The model under review builds one solid part; all positions refer to its coordinate system, in mm. A direction names the side the tool comes from. Round coordinates to 2 decimals unless told otherwise and drop trailing zeros. Write each loop counter-clockwise with the first axis right and the second up, starting at its lowest first coordinate (ties: lowest second). Pieces come first, ordered by that corner, then holes. Notation, with made-up numbers: (62, 6) -> (84, 6) arc R25 cw to (84, 39) -> close; hole circle Ø4 at (87.25, 70). An arc over 180 degrees is marked (long way). Answer in a Markdown table with one row per item. Add a question column.
Autodesk Inventor part; units mm, degrees
ref_plane "YZ Plane" through (0, 0, 0) normal (1, 0, 0) x (0, 1, 0)
ref_plane "XZ Plane" through (0, 0, 0) normal (0, 1, 0) x (-1, 0, 0)
ref_plane "XY Plane" through (0, 0, 0) normal (0, 0, 1) x (1, 0, 0)
sketch "Sketch1" plane through (0, 0, 0) normal (0, 1, 0) x (-1, 0, 0)
  line L0 (0, 0) -> (152.4, 0)
  line L1 (152.4, 0) -> (152.4, 152.4)
  line L2 (152.4, 152.4) -> (0, 152.4)
  line L3 (0, 152.4) -> (0, 0)
  dimension "d0" = 152.4
  dimension "d1" = 152.4
extrude "Extrusion1" add sketch "Sketch1" along normal blind 6.35
sketch "Sketch2" plane through (0, 6.35, 0) normal (0, 1, 0) x (1, 0, 0)
  line L0 (-142.24, -142.24) -> (-77.47, -142.24)
  line L1 (-77.47, -142.24) -> (-77.47, -132.08)
  line L2 (-77.47, -132.08) -> (-142.24, -132.08)
  line L3 (-142.24, -132.08) -> (-142.24, -142.24)
  line L4 (-74.93, -142.24) -> (-10.16, -142.24)
  line L5 (-10.16, -142.24) -> (-10.16, -132.08)
  line L6 (-10.16, -132.08) -> (-74.93, -132.08)
  line L7 (-74.93, -132.08) -> (-74.93, -142.24)
  line L8 (-152.4, 0) -> (-152.4, -152.4)
  line L9 (-152.4, -152.4) -> (0, -152.4)
  line L10 (0, -152.4) -> (0, 0)
  line L11 (-152.4, -76.2) -> (0, -76.2) construction
  line L12 (-142.24, -10.16) -> (-77.47, -10.16)
  line L13 (-77.47, -10.16) -> (-77.47, -20.32)
  line L14 (-77.47, -20.32) -> (-142.24, -20.32)
  line L15 (-142.24, -20.32) -> (-142.24, -10.16)
  line L16 (-74.93, -10.16) -> (-10.16, -10.16)
  line L17 (-10.16, -10.16) -> (-10.16, -20.32)
  line L18 (-10.16, -20.32) -> (-74.93, -20.32)
  line L19 (-74.93, -20.32) -> (-74.93, -10.16)
  point P0 (-10.16, -137.16)
  point P1 (-10.16, -15.24)
  dimension "d4" = 10.16
  dimension "d5" = 10.16
  dimension "d6" = 10.16
  dimension "d7" = 64.77
  dimension "d8" = 64.77
  dimension "d9" = 10.16
  dimension "d10" = 10.16
  dimension "d11" = 10.16
extrude "Extrusion2" cut sketch "Sketch2" against normal through all
sketch "Sketch3" plane through (0, 6.35, 0) normal (0, 1, 0) x (1, 0, 0)
  line L0 (-77.47, -20.32) -> (-142.24, -20.32)
  line L1 (-142.24, -20.32) -> (-142.24, -10.16)
  line L2 (-142.24, -10.16) -> (-77.47, -10.16)
  line L3 (-77.47, -10.16) -> (-77.47, -20.32)
  line L4 (-74.93, -132.08) -> (-10.16, -132.08)
  line L5 (-10.16, -132.08) -> (-10.16, -142.24)
  line L6 (-10.16, -142.24) -> (-74.93, -142.24)
  line L7 (-74.93, -142.24) -> (-74.93, -132.08)
  line L8 (-10.16, -10.16) -> (-10.16, -20.32)
  line L9 (-10.16, -20.32) -> (-74.93, -20.32)
  line L10 (-74.93, -20.32) -> (-74.93, -10.16)
  line L11 (-74.93, -10.16) -> (-10.16, -10.16)
  line L12 (-142.24, -132.08) -> (-77.47, -132.08)
  line L13 (-77.47, -132.08) -> (-77.47, -142.24)
  line L14 (-77.47, -142.24) -> (-142.24, -142.24)
  line L15 (-142.24, -142.24) -> (-142.24, -132.08)
  line L16 (-152.4, 0) -> (-152.4, -152.4)
  line L17 (-152.4, -152.4) -> (0, -152.4)
  line L18 (0, -152.4) -> (0, 0)
  line L19 (0, 0) -> (-152.4, 0)
  line L20 (-146.05, -146.05) -> (-146.05, -6.35)
  line L21 (-146.05, -6.35) -> (-6.35, -6.35)
  line L22 (-6.35, -6.35) -> (-6.35, -146.05)
  line L23 (-6.35, -146.05) -> (-146.05, -146.05)
  dimension "d14" = 6.35
extrude "Extrusion3" add sketch "Sketch3" along normal blind 38.1 contours L19 L18 L17 L16
ref_plane "Work Plane1" through (0, 22.225, 0) normal (0, 1, 0) x (1, 0, 0)
mirror "Mirror1" about plane through (0, 22.225, 0) normal (0, 1, 0) of "Extrusion1", "Extrusion2"
sketch "Sketch5" plane through (0, 22.225, 0) normal (0, 1, 0) x (1, 0, 0)
  line L0 (-142.24, -10.16) -> (-77.47, -10.16)
  line L1 (-77.47, -10.16) -> (-77.47, -20.32)
  line L2 (-77.47, -20.32) -> (-142.24, -20.32)
  line L3 (-142.24, -20.32) -> (-142.24, -10.16)
  line L4 (-142.24, -142.24) -> (-142.24, -132.08)
  line L5 (-142.24, -132.08) -> (-77.47, -132.08)
  line L6 (-77.47, -132.08) -> (-77.47, -142.24)
  line L7 (-77.47, -142.24) -> (-142.24, -142.24)
  line L8 (-74.93, -20.32) -> (-74.93, -10.16)
  line L9 (-74.93, -10.16) -> (-10.16, -10.16)
  line L10 (-10.16, -10.16) -> (-10.16, -20.32)
  line L11 (-10.16, -20.32) -> (-74.93, -20.32)
  line L12 (-74.93, -142.24) -> (-74.93, -132.08)
  line L13 (-74.93, -132.08) -> (-10.16, -132.08)
  line L14 (-10.16, -132.08) -> (-10.16, -142.24)
  line L15 (-10.16, -142.24) -> (-74.93, -142.24)
  line L16 (-152.4, -152.4) -> (0, -152.4)
  line L17 (0, -152.4) -> (0, 0)
  line L18 (0, 0) -> (-152.4, 0)
  line L19 (-152.4, 0) -> (-152.4, -152.4)
extrude "Extrusion4" cut sketch "Sketch5" against normal through all contours L0 L1 L2 L3 | L4 L5 L6 L7 | L8 L9 L10 L11 | L12 L13 L14 L15 | L19 L18 L17 L16
equation "\"d8\" = d7"
equation "\"d10\" = d5"
equation "\"d11\" = d6"
properties part number "Bot v1 top"
1. Add section A-A on x = -139.5. Write out the cut boundary in (y, z) (3 decimals), plus the area to 3 significant figures.
2. Add section D-D on z = 118.5. Write out the cut boundary in (x, y) (3 decimals), plus the area to 3 significant figures.
3. For L1, parallel to Z at x = -86.5, y = 38.25; L2, parallel to X at y = 28.5, z = 60.5; L3, parallel to Z at x = -139, y = 34.25, list the stretches that pass through material, from the lowest coordinate up.
4. Add section B-B on z = 138. Write out the cut boundary in (x, y) (3 decimals).
5. Insertion check: pin 1 Ø4 at (x, z) = (-60.5, 101) entering from -Y. The pin has a flat end and moves straight along its axis. Give the tip position at first contact, or say it passes through.
6. Mouldability with a two-part tool opening along Z and no side actions: class faces 1 (the flat face through (-77, 38.1, 77)), 2 (the flat face through (-77, 44.45, 75)), 3 (the flat face through (-75, 33, 0)) as pulls with the +Z half, pulls with the -Z half, needs draft (parallel to the pull), parting line crosses it, or undercut.
7. Add section C-C on y = 35.5. Write out the cut boundary in (x, z).
8. Tool access review of faces 4 (the flat face through (-152.4, 33, 75)), 5 (the flat face through (-75, 30, 146.05)), 6 (the flat face through (-10.16, 41, 137)): name each direction out of +Z, -Z, +X, -X, +Y, -Y from which nothing blocks a thin tool from reaching the whole face with its end or side.
Filled in:
| question | item | result |
|---|---|---|
| 1 | outline | (22.225, 0) -> (44.45, 0) -> (44.45, 10.16) -> (38.1, 10.16) -> (38.1, 6.35) -> (22.225, 6.35) -> close; (22.225, 146.05) -> (38.1, 146.05) -> (38.1, 142.24) -> (44.45, 142.24) -> (44.45, 152.4) -> (22.225, 152.4) -> close; (38.1, 20.32) -> (44.45, 20.32) -> (44.45, 132.08) -> (38.1, 132.08) -> close |
| 1 | area | 1,040 mm² |
| 2 | outline | (-152.4, 22.225) -> (-146.05, 22.225) -> (-146.05, 38.1) -> (-6.35, 38.1) -> (-6.35, 22.225) -> (0, 22.225) -> (0, 44.45) -> (-152.4, 44.45) -> close |
| 2 | area | 1,170 mm² |
| 3 | L1 | 0 to 10.16, 20.32 to 132.08, 142.24 to 152.4 |
| 3 | L2 | -152.4 to -146.05, -6.35 to 0 |
| 3 | L3 | 0 to 6.35, 146.05 to 152.4 |
| 4 | outline | (-152.4, 22.225) -> (-146.05, 22.225) -> (-146.05, 38.1) -> (-142.24, 38.1) -> (-142.24, 44.45) -> (-152.4, 44.45) -> close; (-77.47, 38.1) -> (-74.93, 38.1) -> (-74.93, 44.45) -> (-77.47, 44.45) -> close; (-10.16, 38.1) -> (-6.35, 38.1) -> (-6.35, 22.225) -> (0, 22.225) -> (0, 44.45) -> (-10.16, 44.45) -> close |
| 5 | pin 1 | y = 38.1 |
| 6 | face 1 | undercut |
| 6 | face 2 | needs draft |
| 6 | face 3 | pulls with the -Z half |
| 7 | outline | (-152.4, 0) -> (0, 0) -> (0, 152.4) -> (-152.4, 152.4) -> close; hole (-146.05, 6.35) -> (-6.35, 6.35) -> (-6.35, 146.05) -> (-146.05, 146.05) -> close |
| 8 | face 4 | +Z, -Z, -X, +Y, -Y |
| 8 | face 5 | -Y |
| 8 | face 6 | +Y, -Y |
